from build123d import *

# Parameters (mm, degrees)
SKETCH1_W           = 104
SKETCH1_H           = 60
SKETCH1_R           = 2.4
BOSS_EXTRUDE1_DEPTH = 6
SKETCH2_W           = 25
SKETCH2_H           = 44
BOSS_EXTRUDE2_DEPTH = 10
SKETCH3_R           = 1.4
CUT_EXTRUDE1_DEPTH  = 11
CHAMFER1_SIZE       = 5


with BuildPart() as part:
    # Sketch1 → Boss-Extrude1 (new body)
    with BuildSketch(Plane(origin=(0, 0, 0), x_dir=(1, 0, 0), z_dir=(0, 1, 0))):
        with Locations((46, 24)):
            Rectangle(SKETCH1_W, SKETCH1_H)
        with Locations((0, 48)):
            Circle(SKETCH1_R, mode=Mode.SUBTRACT)
        with Locations((92, 48)):
            Circle(SKETCH1_R, mode=Mode.SUBTRACT)
        with Locations((92, 0)):
            Circle(SKETCH1_R, mode=Mode.SUBTRACT)
        Circle(SKETCH1_R, mode=Mode.SUBTRACT)
    extrude(amount=BOSS_EXTRUDE1_DEPTH)

    # Sketch2 → Boss-Extrude2 (add)
    with BuildSketch(Plane.XY.offset(6)):
        with Locations((6.5, 28)):
            Rectangle(SKETCH2_W, SKETCH2_H)
    extrude(amount=-BOSS_EXTRUDE2_DEPTH)

    # Sketch3 → Cut-Extrude1 (cut, through all)
    with BuildSketch(Plane(origin=(0, 0, -4), x_dir=(-1, 0, 0), z_dir=(0, 0, -1))):
        with Locations((-15.5, 9.5)):
            Circle(SKETCH3_R)
        with Locations((2.5, 46.5)):
            Circle(SKETCH3_R)
    extrude(amount=-CUT_EXTRUDE1_DEPTH, mode=Mode.SUBTRACT)

    # Chamfer1
    chamfer1_edges = [part.edges().sort_by_distance(p)[0] for p in [
        (19, 50, 1),
    ]]
    chamfer(chamfer1_edges, length=CHAMFER1_SIZE)


solid = part.part
Source: CAD feature listing. Evaluate the final solid. Frame: model axes, mm. A direction names the side the tool comes from. Round coordinates to 2 decimals unless told otherwise and drop trailing zeros. Loops run counter-clockwise (first coordinate to the right, second up) from the corner with the lowest first, then second, coordinate; pieces in that order, holes last. Notation, with made-up numbers: (-12, -7) -> (30, -7) arc R14 ccw to (30, 0) -> close; hole circle Ø6 at (7.25, 52.25). An arc over 180 degrees is marked (long way). Answer as a JSON object with one key per item and string values. Group by question number.
Q1. Mould query, pull axis Y, two halves, no side actions, for faces 4 (the cylindrical face through (16.9, 9.56, 0.93)), 5 (the flat face through (4, 50, 1)), 6 (the flat face through (6, 28, -4)). Classes: pulls with the +Y half, pulls with the -Y half, needs draft (parallel to the pull), parting line crosses it, or undercut.
Q2. Section query B-B (y = 46.5). Output: boundary loops of the cut face in (x, z).
Q3. Section query C-C (z = 0). Output: boundary loops of the cut face in (x, y).
Q4. Section query D-D (z = -48). Output: boundary loops of the cut face in (x, y).
Q5. Contact query for flat-ended pins moving along their axis: P1, Ø12, axis at x = 27, z = -36, coming from the +Y side; P2, Ø3, axis at x = 0, z = -48, coming from the +Y side; P3, Ø6, axis at x = 21.5, y = 13, coming from the -Z side; P4, Ø8, axis at y = 30.5, z = 1, coming from the +X side. Output: stop coordinate, or through.
Q6. Access query for faces 1 (the flat face through (45, 0, -24)), 2 (the flat face through (19, 25, 1)), 3 (the flat face through (0, 6, 0)). Directions: +Z, -Z, +X, -X, +Y, -Y. A direction counts if a zero-diameter tool reaches every point of the face in a straight line with its end or side. Return the directions, or none.
Q7. Section query A-A (x = 15.5). Output: boundary loops of the cut face in (y, z).
Q8. Ray query, line 1 (X direction, y = 1.8, z = 0); line 2 (Z direction, x = 0, y = 1.5); line 3 (Y direction, x = 71.5, z = -32.5). Return the intervals inside material, ascending. Write a range as from..to.
Completed:
{
 "1": {"face 4": "undercut", "face 5": "pulls with the +Y half", "face 6": "needs draft"},
 "2": {"outline": "(-6, -4) -> (-3.9, -4) -> (-3.9, 6) -> (-6, 6) -> close; (-1.1, -4) -> (17.5, -4) -> (17.5, 6) -> (-1.1, 6) -> close"},
 "3": {"outline": "(-6, 0) -> (-2.4, 0) -> (-2.4, 6) -> (2.4, 6) -> (2.4, 0) -> (89.6, 0) -> (89.6, 6) -> (19, 6) -> (19, 45) -> (14, 50) -> (-6, 50) -> close; (94.4, 0) -> (98, 0) -> (98, 6) -> (94.4, 6) -> close; hole circle Ø2.8 at (-2.5, 46.5); hole circle Ø2.8 at (15.5, 9.5)"},
 "4": {"outline": "(-6, 0) -> (-2.4, 0) -> (-2.4, 6) -> (-6, 6) -> close; (2.4, 0) -> (89.6, 0) -> (89.6, 6) -> (2.4, 6) -> close; (94.4, 0) -> (98, 0) -> (98, 6) -> (94.4, 6) -> close"},
 "5": {"P1": "y = 6", "P2": "through", "P3": "z = -4", "P4": "x = 19"},
 "6": {"face 1": "+Z, -Z, +X, -X, -Y", "face 2": "+Z, -Z, +X, +Y", "face 3": "-Y"},
 "7": {"outline": "(0, -54) -> (6, -54) -> (6, -4) -> (8.1, -4) -> (8.1, 6) -> (0, 6) -> close; (10.9, -4) -> (48.5, -4) -> (48.5, 6) -> (10.9, 6) -> close"},
 "8": {"line 1": "-6..-2.4, 2.4..89.6, 94.4..98", "line 2": "-54..-50.4, -45.6..-2.4, 2.4..6", "line 3": "0..6"}
}
